Can you work these out from the drawing? Everything is in mm from the part's minimum corner. Coordinates: 2 decimals unless noted, no trailing zeros. Loops run counter-clockwise (first coordinate to the right, second up) from the corner with the lowest first, then second, coordinate; pieces in that order, holes last.
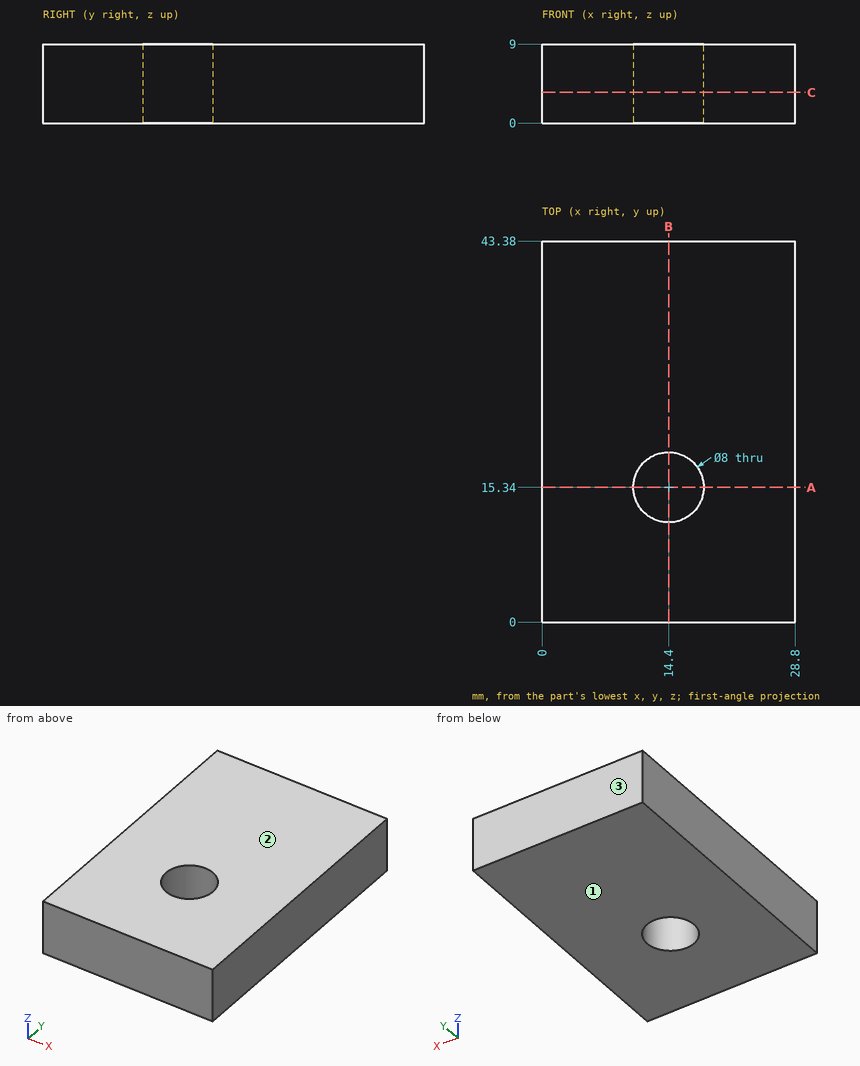
Item 1: We'd pull the mould along Z, two halves only. Please class the marked faces 1, 2 and 3: +Z half, -Z half, draft (parallel to the pull), parting line (faces both ways), or undercut.
Results are:
face 1: -Z half
face 2: +Z half
face 3: draft
Item 2: Suppose I cut it at A-A, the plane y = 15.34. Please give me the cut outline in (x, z), plus the area to 3 significant figures.
Results are:
outline: (0, 0) - (10.4, 0) - (10.4, 9) - (0, 9) - close; (18.4, 0) - (28.8, 0) - (28.8, 9) - (18.4, 9) - close
area: 187 mm2
Item 3: I need wall thicknesses on line 1 along Y through (x, z) = (14.4, 5.25); line 2 along Y through (x, z) = (15.5, 3.5). Which ranges of each line are inside material? Lowest first, please.
Results are:
line 1: y = 0 to 11.34, 19.34 to 43.38
line 2: y = 0 to 11.49, 19.19 to 43.38
Item 4: Suppose I cut it at C-C, the plane z = 3.5. Please give me the cut outline in (x, y).
Results are:
outline: (0, 0) - (28.8, 0) - (28.8, 43.38) - (0, 43.38) - close; hole circle Ø8 at (14.4, 15.34)
Item 5: Suppose I cut it at B-B, the plane x = 14.4. Please give me the cut outline in (y, z).
Results are:
outline: (0, 0) - (11.34, 0) - (11.34, 9) - (0, 9) - close; (19.34, 0) - (43.38, 0) - (43.38, 9) - (19.34, 9) - close
